```python
from build123d import *

# Parameters (mm, degrees)
BASE_FLANGE1_DEPTH           = 3.175
M8_CLEARANCE_HOLE1_D         = 9
EDGE_FLANGE1_DEPTH           = 16.378
EDGE_FLANGE2_STRIP_W         = 14.1732
EDGE_FLANGE2_STRIP_H         = 3.175
EDGE_FLANGE2_STRIP_CUT_DEPTH = 16.378
EDGE_FLANGE2_DEPTH           = 16.378
M5_CLEARANCE_HOLE1_D         = 5.5
FILLET1_R                    = 2.54


# Sheet-metal steps are written as plain solids
with BuildPart() as part:
    # Sketch1 → Base-Flange1 (new body)
    with BuildSketch(Plane.XY):
        Polygon((0, 0), (57.15, 0), (57.15, -16.378), (57.15, -22.8346), (61.9125, -22.8346), (61.9125, -39.2126), (57.15, -39.2126), (40.772, -39.2126), (40.772, -16.378), (0, -16.378), align=None)
    extrude(amount=-BASE_FLANGE1_DEPTH)

    # M8 Clearance Hole1 (through all)
    with Locations(Plane.XY):
        with Locations((10, -8.189)):
            Hole(M8_CLEARANCE_HOLE1_D / 2)

    # Edge-Flange1 section (across the edge) → Edge-Flange1 (add)
    with BuildSketch(Plane(origin=(62.6491, -39.2126, 0), x_dir=(-1, 0, 0), z_dir=(0, 1, 0))):
        with BuildLine():
            Line((-3.175, 0.7366), (-3.175, 23.9268))
            Line((-3.175, 23.9268), (0, 23.9268))
            Line((0, 23.9268), (0, 0.7366))
            ThreePointArc((0, 0.7366), (0.215745145, 0.215745145), (0.7366, 0))
            Line((0.7366, 0), (0.7366, -3.175))
            ThreePointArc((0.7366, -3.175), (-2.029318885, -2.029318885), (-3.175, 0.7366))
        make_face()
    extrude(amount=EDGE_FLANGE1_DEPTH)

    # Edge-Flange2 strip (across the edge) → Edge-Flange2 strip cut (cut)
    with BuildSketch(Plane(origin=(65.8241, -22.8346, 23.9268), x_dir=(0, 0, -1), z_dir=(0, -1, 0))):
        with Locations((-6.35, -1.5875)):
            Rectangle(EDGE_FLANGE2_STRIP_W, EDGE_FLANGE2_STRIP_H)
    extrude(amount=EDGE_FLANGE2_STRIP_CUT_DEPTH, mode=Mode.SUBTRACT)

    # Edge-Flange2 section (across the edge) → Edge-Flange2 (add)
    with BuildSketch(Plane(origin=(65.8241, -22.8346, 23.9268), x_dir=(0, 0, -1), z_dir=(0, -1, 0))):
        with BuildLine():
            Line((-3.175, 0.7366), (-3.175, 34.925))
            Line((-3.175, 34.925), (0, 34.925))
            Line((0, 34.925), (0, 0.7366))
            ThreePointArc((0, 0.7366), (0.215745145, 0.215745145), (0.7366, 0))
            Line((0.7366, 0), (0.7366, -3.175))
            ThreePointArc((0.7366, -3.175), (-2.029318885, -2.029318885), (-3.175, 0.7366))
        make_face()
    extrude(amount=EDGE_FLANGE2_DEPTH)

    # M5 Clearance Hole1 (through all)
    with Locations(Plane.XY.offset(27.1018)):
        with Locations((94.9349, -31.0236)):
            Hole(M5_CLEARANCE_HOLE1_D / 2)

    # Fillet1
    fillet1_edges = [part.edges().sort_by_distance(p)[0] for p in [
        (0, 0, -1.5875),
        (57.15, 0, -1.5875),
        (57.15, -22.8346, -1.5875),
        (40.772, -39.2126, -1.5875),
        (40.772, -16.378, -1.5875),
        (0, -16.378, -1.5875),
        (100.7491, -22.8346, 25.5143),
        (100.7491, -39.2126, 25.5143),
    ]]
    fillet(fillet1_edges, radius=FILLET1_R)


solid = part.part
```
Geometry: final body of the model. Coordinates: model frame, mm. A direction names the side the tool comes from. Coordinates: 2 decimals unless noted, no trailing zeros. Write each loop counter-clockwise with the first axis right and the second up, starting at its lowest first coordinate (ties: lowest second). Pieces come first, ordered by that corner, then holes. Notation, with made-up numbers: M 48.5,25 L 52.5,25 A26 cw 52.5,64 Z; hole C 8.25,-27.75 d10. An arc over 180 degrees is marked long. Use CSV: the item, a comma, the result in double quotes. Start each with the question number.
1. Reachability of faces 4 (the face through (65.824, -31, 12)), 5 (the face through (62.649, -31, 12)), 6 (the face through (21, -16.378, -2)) from +Z, -Z, +X, -X, +Y, -Y: full face, straight path, thin tool, end or side. Return the list, or none.
2. Cut plane C-C on z = 2. Return the cut outline in (x, y), plus the area to 3 significant figures.
3. Ray query, probe 1 along Y at (x, z) = (10, -1.35); probe 2 along X at (y, z) = (-31.5, 8); probe 3 along Z at (x, y) = (42, -21) (3 decimals). Return the intervals inside material, ascending.
4. Cut plane D-D on y = -29.5. Return the cut outline in (x, z) (1 decimal), plus the area to 3 significant figures.
5. Cut plane A-A on x = 10. Return the cut outline in (y, z) (3 decimals).
6. Mould query, pull axis X, two halves, no side actions, for faces 1 (the face through (0.764, -0.724, -1.61)), 2 (the face through (57.15, -12, -2)), 3 (the face through (5.708, -6.837, -1.61)). Classes: pulls with the +X half, pulls with the -X half, needs draft (parallel to the pull), parting line crosses it, or undercut.
7. First-contact query: P1, Ø2.5, axis at x = 19, z = -2, coming from the -Y side; P2, Ø5, axis at y = -28.5, z = 12.5, coming from the -X side; P3, Ø9, axis at x = 94.93, y = -31.02, coming from the -Z side; P4, Ø15, axis at x = 74.5, z = 10.5, coming from the +Y side. Flat tips, straight axial feed; report the tip coordinate or a pass-through.
8. Cut plane B-B on y = -6. Return the cut outline in (x, z) (3 decimals), plus the area to 3 significant figures.
Entries:
1,face 4,"-Z, +X, +Y, -Y"
1,face 5,"+Z, -X, +Y, -Y"
1,face 6,"+Z, -Z, -X, -Y"
2,outline,"M 62.65,-39.21 L 65.82,-39.21 L 65.82,-22.83 L 62.65,-22.83 Z"
2,area,"52.0 mm²"
3,probe 1,"-16.38 to -12.69, -3.69 to 0"
3,probe 2,"62.65 to 65.82"
3,probe 3,"-3.175 to 0"
4,outline,"M 40.8,-3.2 L 61.9,-3.2 A3.9 ccw 65.8,0.7 L 65.8,23.2 A0.7 cw 66.6,23.9 L 92.6,23.9 L 92.6,27.1 L 66.6,27.1 A3.9 ccw 62.6,23.2 L 62.6,0.7 A0.7 cw 61.9,0 L 40.8,0 Z; M 97.2,23.9 L 100.7,23.9 L 100.7,27.1 L 97.2,27.1 Z"
4,area,"256 mm²"
5,outline,"M -16.378,-3.175 L -12.689,-3.175 L -12.689,0 L -16.378,0 Z; M -3.689,-3.175 L 0,-3.175 L 0,0 L -3.689,0 Z"
6,face 1,"pulls with the -X half"
6,face 2,"pulls with the +X half"
6,face 3,"undercut"
7,P1,"y = -16.38"
7,P2,"x = 62.65"
7,P3,"z = 23.93"
7,P4,"through"
8,outline,"M 0,-3.175 L 6.068,-3.175 L 6.068,0 L 0,0 Z; M 13.932,-3.175 L 57.15,-3.175 L 57.15,0 L 13.932,0 Z"
8,area,"156 mm²"
